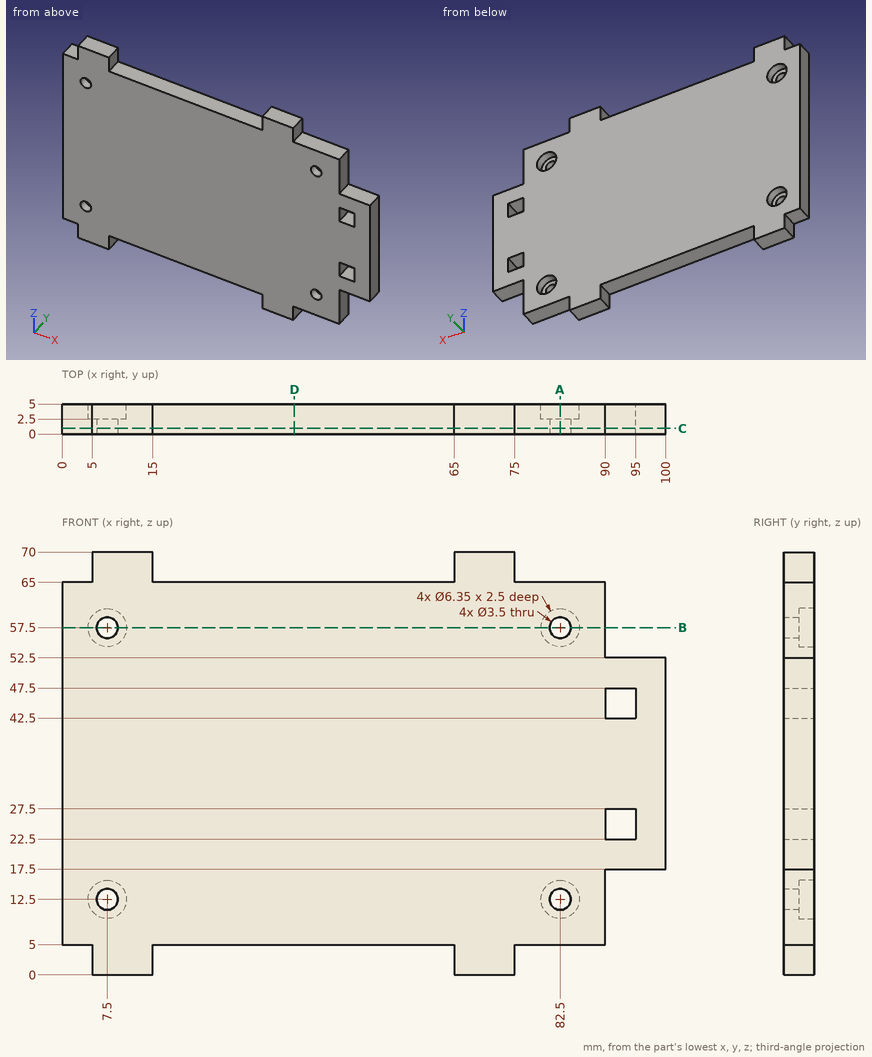
Can you work these out from the drawing? Everything is in mm from the part's minimum corner. Give positions to 0.01 mm unless a question says otherwise; leave off trailing zeros. Loops run counter-clockwise (first coordinate to the right, second up) from the corner with the lowest first, then second, coordinate; pieces in that order, holes last. Notation, with made-up numbers: (-34.5, 4.25) - (-27.5, 4.25) arc R10 ccw to (-27.5, 13.25) - close; hole circle Ø2 at (53.25, 22.25). An arc over 180 degrees is marked (long way). Use one line per item in the form item = value.
1. I want a section at D-D (x = 38.5). Please give me the cut outline in (y, z).
Response values:
outline = (0, 5) - (5, 5) - (5, 65) - (0, 65) - close
2. I want a section at C-C (y = 0.95). Give the number of separate pieces and of enclosed holes in the cut face, and give its area (3 significant figures).
Response values:
separate_pieces = 1
enclosed_holes = 6
area = 5,860 mm²
3. I want a section at A-A (x = 82.5). Please give me the cut outline in (y, z) (3 decimals), and give its area (3 significant figures).
Response values:
outline = (0, 5) - (5, 5) - (5, 9.325) - (2.5, 9.325) - (2.5, 10.75) - (0, 10.75) - close; (0, 14.25) - (2.5, 14.25) - (2.5, 15.675) - (5, 15.675) - (5, 54.325) - (2.5, 54.325) - (2.5, 55.75) - (0, 55.75) - close; (0, 59.25) - (2.5, 59.25) - (2.5, 60.675) - (5, 60.675) - (5, 65) - (0, 65) - close
area = 251 mm²
4. I want a section at B-B (z = 57.5). Please give me the cut outline in (x, y) (3 decimals), and give its area (3 significant figures).
Response values:
outline = (0, 0) - (5.75, 0) - (5.75, 2.5) - (4.325, 2.5) - (4.325, 5) - (0, 5) - close; (9.25, 0) - (80.75, 0) - (80.75, 2.5) - (79.325, 2.5) - (79.325, 5) - (10.675, 5) - (10.675, 2.5) - (9.25, 2.5) - close; (84.25, 0) - (90, 0) - (90, 5) - (85.675, 5) - (85.675, 2.5) - (84.25, 2.5) - close
area = 401 mm²
5. I'm going to push flat-ended pins straight in: pin 1 Ø1.9 at (x, z) = (8.5, 59) entering from +Y; pin 2 Ø3 at (x, z) = (82.5, 57.5) entering from -Y; pin 3 Ø2 at (x, y) = (19.5, 4) entering from +Z; pin 4 Ø2.5 at (x, y) = (91.5, 3.5) entering from -Z. Where does each tip first touch, or does it pass through?
Response values:
pin_1 = 2.5
pin_2 = through
pin_3 = 65
pin_4 = 17.5
6. I need wall thicknesses on probe 1 along Z at (x, y) = (7.5, 1.3); probe 2 along X at (y, z) = (3.7, 12.5) (3 decimals); probe 3 along X at (y, z) = (1.15, 57.5). Which ranges of each line are inside material? Lowest first, please.
Response values:
probe_1 = 0 to 10.75, 14.25 to 55.75, 59.25 to 70
probe_2 = 0 to 4.325, 10.675 to 79.325, 85.675 to 90
probe_3 = 0 to 5.75, 9.25 to 80.75, 84.25 to 90
